Here's the drawing with two shaded views (mm, measured from the low corner). I have some questions. Round coordinates to 2 decimals unless told otherwise and drop trailing zeros. Order: outer loops, then holes, each group sorted by start corner. A loop starts at its lowest first (then second) coordinate and runs counter-clockwise, first axis right, second up.
Q1. If we section it at A-A (x = 342.9): Please give me the cut outline in (y, z).
Q2. If we section it at C-C (y = 75): Please give me the cut outline in (x, z), plus the area to 3 significant figures.
Q3. Will these pins go through, and if not, where does the flat tip stop? P1, Ø8, axis at x = 147, y = 52.5, coming from the +Z side; P2, Ø12, axis at x = 499.5, y = 91.5, coming from the -Z side; P3, Ø2, axis at y = 83, z = 201, coming from the +X side.
Q4. If I drill on line 1 (Z direction, x = 342.9, y = 77.5); line 2 (Z direction, x = 342.9, y = 118.5), over which ranges is the centre line in solid material (lowest first)?
Q5. If we section it at D-D (y = 23): Please give me the cut outline in (x, z).
Q6. We'd pull the mould along Z, two halves only. Please class the marked faces 1 and 2: pulls with the +Z half, pulls with the -Z half, needs draft (parallel to the pull), parting line crosses it, or undercut.
Q7. If we section it at B-B (z = 342.9): Please give me the cut outline in (x, y).
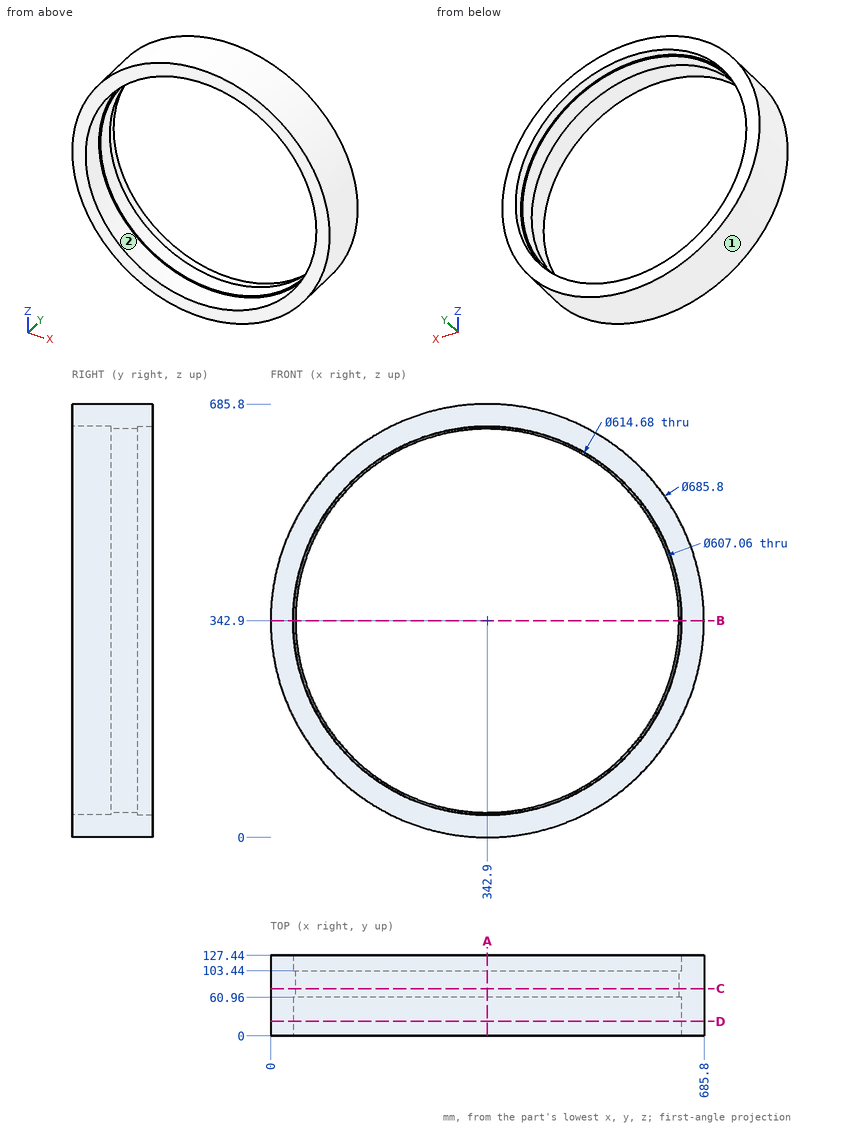
Solution:
1. outline: (0, 0) - (127.44, 0) - (127.44, 35.56) - (103.44, 35.56) - (103.44, 39.37) - (60.96, 39.37) - (60.96, 35.56) - (0, 35.56) - close; (0, 650.24) - (60.96, 650.24) - (60.96, 646.43) - (103.44, 646.43) - (103.44, 650.24) - (127.44, 650.24) - (127.44, 685.8) - (0, 685.8) - close
2. outline: circle Ø685.8 at (342.9, 342.9); hole circle Ø607.06 at (342.9, 342.9)
2. area: 80,000 mm2
3. P1: stops at z = 627.07
3. P2: stops at z = 34.84
3. P3: stops at x = 655.51
4. line 1: z = 0 to 39.37, 646.43 to 685.8
4. line 2: z = 0 to 35.56, 650.24 to 685.8
5. outline: circle Ø685.8 at (342.9, 342.9); hole circle Ø614.68 at (342.9, 342.9)
6. face 1: parting line crosses it
6. face 2: undercut
7. outline: (0, 0) - (35.56, 0) - (35.56, 60.96) - (39.37, 60.96) - (39.37, 103.44) - (35.56, 103.44) - (35.56, 127.44) - (0, 127.44) - close; (646.43, 60.96) - (650.24, 60.96) - (650.24, 0) - (685.8, 0) - (685.8, 127.44) - (650.24, 127.44) - (650.24, 103.44) - (646.43, 103.44) - close
